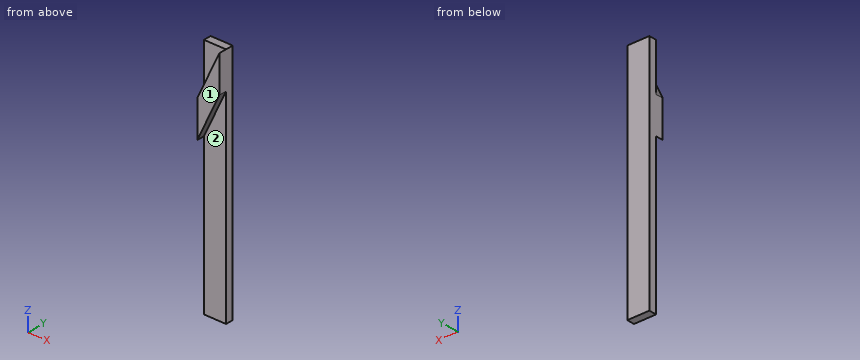
```python
from build123d import *

# Parameters (mm, degrees)
BOSS_EXTRUDE1_DEPTH = 5
BOSS_EXTRUDE2_START = -5
BOSS_EXTRUDE2_DEPTH = 5


# Read off the part's stored shape, not the designer's step: Boss-Extrude2
with BuildPart() as part:
    # Sketch1 → Boss-Extrude1 (new body)
    with BuildSketch(Plane(origin=(0, 0, 0), x_dir=(1, 0, 0), z_dir=(0, 1, 0))):
        Polygon((14.359671821, -155.090990788), (0, -124.296575192), (0, -155.090990788), align=None)
        Polygon((0, -100.63455936), (0, -124.296575192), (14.359671821, -155.090990788), (14.359671821, -131.428974957), align=None)
        Polygon((0, 0), (0, -100.63455936), (14.359671821, -131.428974957), (14.359671821, 0), align=None)
    extrude(amount=BOSS_EXTRUDE1_DEPTH)

    # Boss-Extrude2 outline → Boss-Extrude2 (add)
    with BuildSketch(Plane(origin=(0, 0, 0), x_dir=(1, 0, 0), z_dir=(0, 1, 0)).offset(BOSS_EXTRUDE2_START)):
        Polygon((0, -100.63455936), (0, -124.296575192), (14.359671821, -155.090990788), (14.359671821, -131.428974957), align=None)
    extrude(amount=BOSS_EXTRUDE2_DEPTH)


solid = part.part
```
Model file for the job. Use its own axes, mm. Face numbers are marked on the shaded views. A direction names the side the tool comes from. Coordinates: 2 decimals unless noted, no trailing zeros. Order: outer loops, then holes, each group sorted by start corner. A loop starts at its lowest first (then second) coordinate and runs counter-clockwise, first axis right, second up. Notation, with made-up numbers: (-27.5, 86.5) - (-0.5, 86.5) arc R26 ccw to (-0.5, 116.5) - close; hole circle Ø11 at (32, -5). An arc over 180 degrees is marked (long way). Return JSON: item names as keys, results as strings. Group by question number.
1) Saw through at C-C, the plane z = 95. Write the cut outline in (x, y), plus the area to 3 significant figures.
2) Probe line 1 (Y direction, x = 9.75, z = 72); line 2 (Z direction, x = 1.25, y = -4); line 3 (Z direction, x = 9.5, y = -0.75). List the from-to ranges inside material, lowest first. Write a range as from..to.
3) Flat gauge pins, fed straight in: P1, Ø3, axis at x = 7.5, z = 24, coming from the -Y side; P2, Ø5, axis at x = 5, y = -3.5, coming from the +Z side. Where does each tip first touch, or does it go through?
4) Saw through at A-A, the plane z = 126.5. Write the cut outline in (x, y).
5) Tool access for the marked faces 1 and 2: list every direction of +Z, -Z, +X, -X, +Y, -Y with a clear straight run to the whole face (end or side of a thin tool).
6) Saw through at B-B, the plane x = 1.5. Write the cut outline in (y, z), plus the area to 3 significant figures.
Values found:
{
 "1": {"outline": "(0, 0) - (14.36, 0) - (14.36, 5) - (0, 5) - close", "area": "71.8 mm²"},
 "2": {"line 1": "y = 0..5", "line 2": "z = 103.32..126.98", "line 3": "z = 121.01..144.67"},
 "3": {"P1": "stops at y = 0", "P2": "stops at z = 140.38"},
 "4": {"outline": "(0, 0) - (1.03, 0) - (1.03, -5) - (12.06, -5) - (12.06, 0) - (14.36, 0) - (14.36, 5) - (0, 5) - close"},
 "5": {"face 1": "+Z, -Z, +X, -X, -Y", "face 2": "-Z, +X, -Y"},
 "6": {"outline": "(-5, 103.85) - (0, 103.85) - (0, 0) - (5, 0) - (5, 155.09) - (0, 155.09) - (0, 127.51) - (-5, 127.51) - close", "area": "894 mm²"}
}
